```python
from build123d import *

# Parameters (mm, degrees)
SKETCH1_R           = 25.4
BOSS_EXTRUDE1_DEPTH = 91.44
CUT_EXTRUDE1_REACH  = 109.643
SKETCH2_W           = 10.795
SKETCH2_H           = 25.4


with BuildPart() as part:
    # Sketch1 → Boss-Extrude1 (new body)
    with BuildSketch(Plane(origin=(0, 0, 0), x_dir=(1, 0, 0), z_dir=(0, 1, 0))):
        with Locations(Location((0, 0, 0), (0, 0, 270))):
            Circle(SKETCH1_R)
    extrude(amount=BOSS_EXTRUDE1_DEPTH)

    # Sketch2 → Cut-Extrude1 (cut, up to next)
    with BuildSketch(Plane(origin=(25.4, 0, 0), x_dir=(0, 0, -1), z_dir=(1, 0, 0)), mode=Mode.PRIVATE) as cut_extrude1_sk1:
        with Locations((-20.0025, 78.74)):
            Rectangle(SKETCH2_W, SKETCH2_H)
    cut_extrude1_tool1 = extrude(cut_extrude1_sk1.sketch, amount=-CUT_EXTRUDE1_REACH, mode=Mode.PRIVATE) & part.part
    # Sketch2 → Cut-Extrude1 (cut, up to next)
    with BuildSketch(Plane(origin=(25.4, 0, 0), x_dir=(0, 0, -1), z_dir=(1, 0, 0)), mode=Mode.PRIVATE) as cut_extrude1_sk2:
        with Locations((20.0025, 78.74)):
            Rectangle(SKETCH2_W, SKETCH2_H)
    cut_extrude1_tool2 = extrude(cut_extrude1_sk2.sketch, amount=-CUT_EXTRUDE1_REACH, mode=Mode.PRIVATE) & part.part
    add(cut_extrude1_tool1.solids().sort_by_distance((25.4, 78.74, 20.0025))[0], mode=Mode.SUBTRACT)
    add(cut_extrude1_tool2.solids().sort_by_distance((25.4, 78.74, -20.0025))[0], mode=Mode.SUBTRACT)


solid = part.part
```
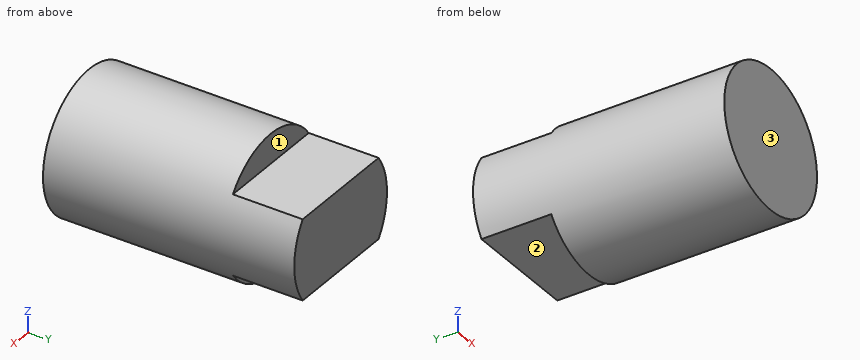
Could you check a few things on this model? Use its own coordinates, in mm. Face numbers are marked on the shaded views. A direction names the side the tool comes from. Give positions to 0.01 mm unless a question says otherwise; leave off trailing zeros. Write each loop counter-clockwise with the first axis right and the second up, starting at its lowest first coordinate (ties: lowest second). Pieces come first, ordered by that corner, then holes. Notation, with made-up numbers: (32, 50) - (75, 50) arc R27 ccw to (75, 85) - close; hole circle Ø9 at (-8.5, 83.5). An arc over 180 degrees is marked (long way). One line per item, written item: value. Start each with the question number.
Item 1: Imagine slicing it at D-D, the plane x = 5.5. List the corners of the cut face in (y, z) for me (3 decimals), and give its area (3 significant figures).
Item 2: Please list where these lines run through material, in increasing order: line 1 (Z direction, x = 1, y = 52); line 2 (Y direction, x = -15, z = -15); line 3 (Z direction, x = -11, y = 67) (3 decimals). Write a range as from..to.
Item 3: I'm going to push flat-ended pins straight in: pin 1 (2 mm diameter, centred on x = 12.5, y = 72, fed in from -Z) (3 decimals); pin 2 (8.5 mm diameter, centred on x = 3, z = -22, fed in from +Y); pin 3 (1.5 mm diameter, centred on x = -17.5, y = 9, fed in from -Z). Where does each tip first touch, or does it pass through?
Item 4: Imagine slicing it at B-B, the plane y = 69. List the corners of the cut face in (x, z) for me (3 decimals).
Item 5: Imagine slicing it at A-A, the plane x = 0. List the corners of the cut face in (y, z) for me (3 decimals), and give its area (3 significant figures).
Item 6: Imagine slicing it at C-C, the plane z = -16. List the corners of the cut face in (x, y) for me, and give its area (3 significant figures).
Item 7: Which directions (+Z, -Z, +X, -X, +Y, -Y) give clear straight access to the entire face, cutting with the end or side of a thin tool? Please do the marked faces 1, 2 and 3.
Geometry says:
1. outline: (0, -24.797) - (66.04, -24.797) - (66.04, -14.605) - (91.44, -14.605) - (91.44, 14.605) - (66.04, 14.605) - (66.04, 24.797) - (0, 24.797) - close
1. area: 4,020 mm^2
2. line 1: -25.38..25.38
2. line 2: 0..66.04
2. line 3: -14.605..14.605
3. pin 1: z = -14.605
3. pin 2: y = 66.04
3. pin 3: z = -19.09
4. outline: (-20.781, -14.605) - (20.781, -14.605) arc R25.4 ccw to (20.781, 14.605) - (-20.781, 14.605) arc R25.4 ccw to start
5. outline: (0, -25.4) - (66.04, -25.4) - (66.04, -14.605) - (91.44, -14.605) - (91.44, 14.605) - (66.04, 14.605) - (66.04, 25.4) - (0, 25.4) - close
5. area: 4,100 mm^2
6. outline: (-19.73, 0) - (19.73, 0) - (19.73, 66.04) - (-19.73, 66.04) - close
6. area: 2,610 mm^2
7. face 1: +Z, +X, -X, +Y
7. face 2: -Z, +X, -X, +Y
7. face 3: +Z, -Z, +X, -X, -Y
